The drawing under review shows one solid part. Ordinate dimensions are in mm from its lowest x, y, z. Give positions to 0.01 mm unless a question says otherwise; leave off trailing zeros. Write each loop counter-clockwise with the first axis right and the second up, starting at its lowest first coordinate (ties: lowest second). Pieces come first, ordered by that corner, then holes.
Q1. Insertion check: P1, Ø6, axis at x = 17, z = 3.5, coming from the -Y side. The pin has a flat end and moves straight along its axis. Give the tip position at first contact, or say it passes through.
Q2. We need section A-A (z = 15.3). Write out the cut boundary in (x, y), then the cut area to 3 significant figures.
Q3. For line 1 (X direction, y = 0.6, z = 1.7); line 2 (X direction, y = 0.2, z = 5), list the stretches that pass through material, from the lowest coordinate up.
Q4. We need section B-B (z = 1.5). Write out the cut boundary in (x, y).
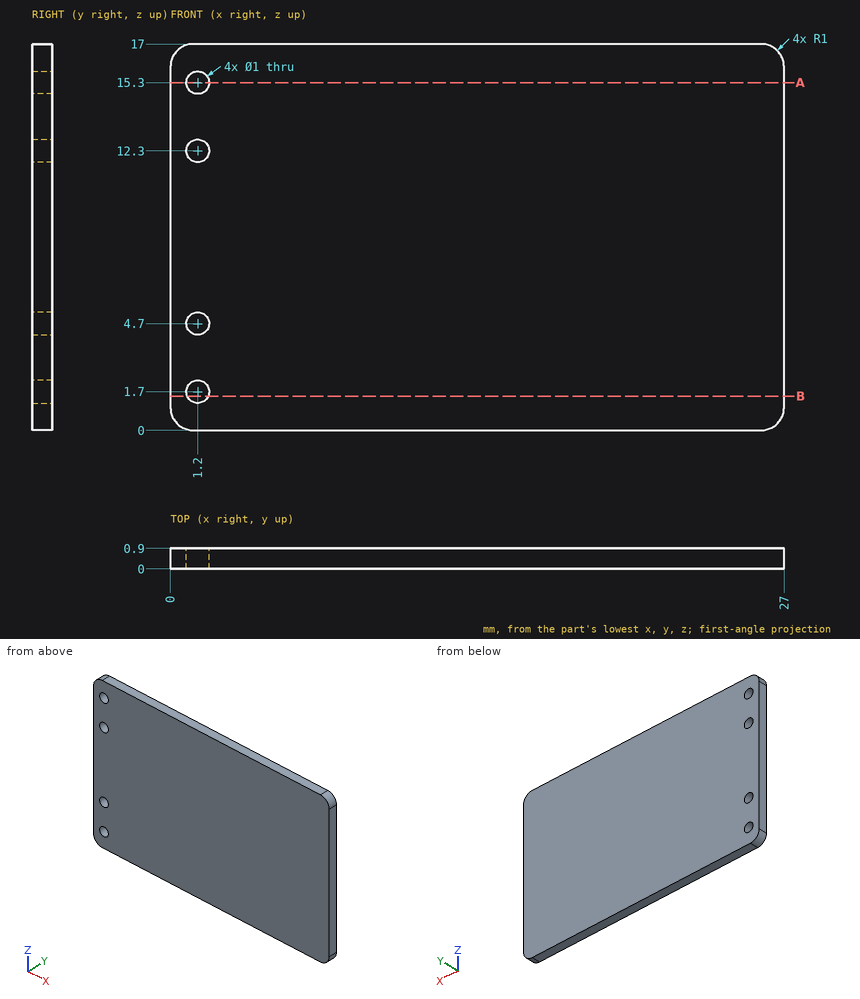
Computed:
1. P1: stops at y = 0
2. outline: (0, 0) - (0.7, 0) - (0.7, 0.9) - (0, 0.9) - close; (1.7, 0) - (27, 0) - (27, 0.9) - (1.7, 0.9) - close
2. area: 23.4 mm2
3. line 1: x = 0 to 0.7, 1.7 to 27
3. line 2: x = 0 to 0.8, 1.6 to 27
4. outline: (0, 0) - (0.74, 0) - (0.74, 0.9) - (0, 0.9) - close; (1.66, 0) - (27, 0) - (27, 0.9) - (1.66, 0.9) - close
